Design review of the part built by this model. Coordinates are the model's own, in mm. Face numbers are marked on the shaded views. Coordinates: 2 decimals unless noted, no trailing zeros. Write each loop counter-clockwise with the first axis right and the second up, starting at its lowest first coordinate (ties: lowest second). Pieces come first, ordered by that corner, then holes. Notation, with made-up numbers: (-3.5, 0.5) -> (39.5, 0.5) arc R13 ccw to (39.5, 15.5) -> close; hole circle Ø4 at (15.5, 12). An arc over 180 degrees is marked (long way). Answer in a Markdown table with one row per item. Add a question column.
Item 1: Clearance check with flat-ended pins moving along their axes: P1, Ø4, axis at x = -29.5, z = 20.5, coming from the -Y side; P2, Ø6, axis at x = 7.5, y = 1252.5, coming from the -Z side; P3, Ø2, axis at x = 5, y = 913, coming from the -Z side. State where each tip first meets the part, or that it passes through.
Item 2: Take a section at C-C, the plane y = 1004. Write out the cut boundary in (x, z).
Item 3: Draft analysis for pull direction Z (two halves, no side actions). For the marked faces 1 and 2, state which applies: released by +Z, released by -Z, zero draft, split by the parting line, or undercut.
Item 4: Take a section at B-B, the plane z = 23.5. Write out the cut boundary in (x, y), and give its area (3 significant figures).
Item 5: Take a section at A-A, the plane x = 0. Write out the cut boundary in (y, z), and give its area (3 significant figures).
Item 6: To check wall thickness, follow line 1 (X direction, y = 399, z = 0); line 2 (X direction, y = 553.5, z = 5). State the ranges of each line that lie inside material, in increasing order.
from build123d import *

# Parameters (mm, degrees)
ESBO_O2_W                  = 39.3
ESBO_O2_H                  = 1640
CORTE_EXTRUS_O1_DEPTH      = 1641.941491949
CORTE_EXTRUS_O1_DEPTH_BACK = 1641.941491949
ESBO_O9_R                  = 35.87378144
CORTE_EXTRUS_O6_DEPTH      = 1641.941491949


with BuildPart() as part:
    # Esboço2 → Revolução2 (revolve)
    with BuildSketch(Plane.XY):
        with Locations((19.65, 820)):
            Rectangle(ESBO_O2_W, ESBO_O2_H)
    revolve(axis=Axis((0, 0, 0), (0, 1, 0)))

    # Esboço3 → Corte-extrusão1 (cut, two sides: drawn at the far end of the back side and taken through both)
    with BuildSketch(Plane.XY.offset(-CORTE_EXTRUS_O1_DEPTH_BACK)):
        Polygon((-39.3, 1640), (39.3, 1640), (-39.3, 1561.4), align=None)
        Polygon((39.3, 0), (-39.3, 78.6), (-39.3, 0), align=None)
    extrude(amount=CORTE_EXTRUS_O1_DEPTH + CORTE_EXTRUS_O1_DEPTH_BACK, mode=Mode.SUBTRACT)

    # Esboço9 → Corte-extrusão6 (cut, through all)
    with BuildSketch(Plane(origin=(0, 0, 0), x_dir=(1, 0, 0), z_dir=(0, 1, 0))):
        Circle(ESBO_O9_R)
    extrude(amount=CORTE_EXTRUS_O6_DEPTH, mode=Mode.SUBTRACT)


solid = part.part
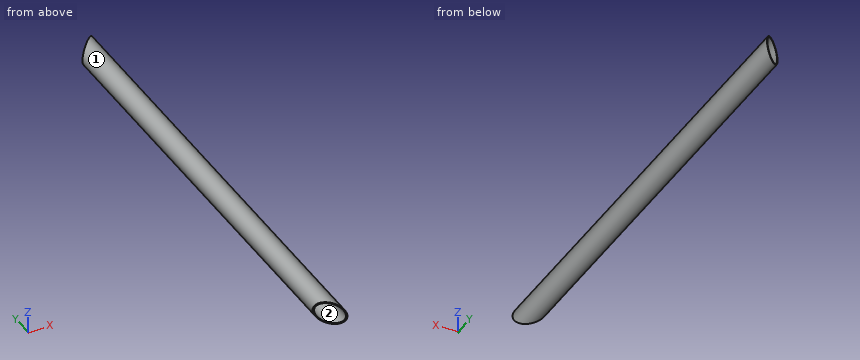
Answers:
| question | item | result |
|---|---|---|
| 1 | P1 | stops at y = 67.57 |
| 1 | P2 | stops at z = -39.04 |
| 1 | P3 | stops at z = -39.1 |
| 2 | outline | circle Ø78.6 at (0, 0); hole circle Ø71.75 at (0, 0) |
| 3 | face 1 | split by the parting line |
| 3 | face 2 | undercut |
| 4 | outline | (-31.5, 70.8) -> (-27.1, 66.4) -> (-27.1, 1573.6) -> (-31.5, 1569.2) -> close; (27.1, 12.2) -> (31.5, 7.8) -> (31.5, 1632.2) -> (27.1, 1627.8) -> close |
| 4 | area | 13,700 mm^2 |
| 5 | outline | (39.3, -39.3) -> (1600.7, -39.3) -> (1600.7, -35.87) -> (39.3, -35.87) -> close; (39.3, 35.87) -> (1600.7, 35.87) -> (1600.7, 39.3) -> (39.3, 39.3) -> close |
| 5 | area | 10,700 mm^2 |
| 6 | line 1 | x = -39.3 to -35.87, 35.87 to 39.3 |
| 6 | line 2 | x = -38.98 to -35.52, 35.52 to 38.98 |
